from build123d import *

# Parameters (mm, degrees)
SKETCH1_W          = 6.35
SKETCH1_H          = 12.7
FILLET1_R          = 3.81
SKETCH2_R          = 2.032
CUT_EXTRUDE1_DEPTH = 5.08


with BuildPart() as part:
    # Sketch1 → Revolve3 (revolve)
    with BuildSketch(Plane.XY, mode=Mode.PRIVATE) as revolve3_sk:
        with Locations((-3.175, 6.35)):
            Rectangle(SKETCH1_W, SKETCH1_H)
    revolve(revolve3_sk.sketch.rotate(Axis((0, -6.586539343, 0), (0, 1, 0)), 270), axis=Axis((0, -6.586539343, 0), (0, 1, 0)))

    # Fillet1
    fillet1_edges = [part.edges().sort_by_distance(p)[0] for p in [
        (0, 12.7, 6.35),
    ]]
    fillet(fillet1_edges, radius=FILLET1_R)

    # Sketch2 → Cut-Extrude1 (cut)
    with BuildSketch(Plane(origin=(0, 0, 0), x_dir=(-1, 0, 0), z_dir=(0, -1, 0))):
        with Locations(Location((0, 0, 0), (0, 0, 90))):
            Circle(SKETCH2_R)
    extrude(amount=-CUT_EXTRUDE1_DEPTH, mode=Mode.SUBTRACT)


solid = part.part
Model file for the job. Use its own axes, mm. A direction names the side the tool comes from. Round coordinates to 2 decimals unless told otherwise and drop trailing zeros. Order: outer loops, then holes, each group sorted by start corner. A loop starts at its lowest first (then second) coordinate and runs counter-clockwise, first axis right, second up.
(1) Band-saw the part on B-B (y = 7.5). List the corners of the cut face in (x, z).
(2) Band-saw the part on A-A (y = 4.5). List the corners of the cut face in (x, z).
(3) 3-axis set-ups, long thin cutter, end or side, ignore diameter. For faces 1 (the face through (0, 5.08, 0)), 2 (the face through (3.86, 4.51, 5.04)): which of +Z, -Z, +X, -X, +Y, -Y reach the whole face in a straight line?
(4) Pin check, flat tips, straight feed: pin 1 (2 mm diameter, centred on x = -4, z = -5, fed in from -Y); pin 2 (2 mm diameter, centred on y = 11, z = 2, fed in from +X); pin 3 (6 mm diameter, centred on x = 4, y = 10, fed in from +Z); pin 4 (1.5 mm diameter, centred on x = 1, y = 5.5, fed in from +Z). Stop position of each tip, or through.
(5) Drill centre lines: line 1 (X direction, y = 3.05, z = 0); line 2 (Y direction, x = 1.5, z = 0.5); line 3 (Z direction, x = -2.5, y = 4.25). Where is each one in solid material? Low to high.
Verdict:
1. outline: circle Ø12.7 at (0, 0)
2. outline: circle Ø12.7 at (0, 0); hole circle Ø4.06 at (0, 0)
3. face 1: -Y
3. face 2: +Y, -Y
4. pin 1: stops at y = 0
4. pin 2: stops at x = 5.96
4. pin 3: stops at z = 6.24
4. pin 4: stops at z = 6.35
5. line 1: x = -6.35 to -2.03, 2.03 to 6.35
5. line 2: y = 5.08 to 12.7
5. line 3: z = -5.84 to 5.84
